Autodesk Inventor part; units mm, degrees
ref_plane "YZ Plane" through (0, 0, 0) normal (1, 0, 0) x (0, 1, 0)
ref_plane "XZ Plane" through (0, 0, 0) normal (0, 1, 0) x (-1, 0, 0)
ref_plane "XY Plane" through (0, 0, 0) normal (0, 0, 1) x (1, 0, 0)
sketch "Sketch1" plane through (0, 0, 0) normal (0, 0, 1) x (1, 0, 0)
  line L0 (-106.553, -66.04) -> (-3.175, -66.04)
  line L1 (0, -62.865) -> (0, -3.175)
  line L2 (-3.175, 0) -> (-106.553, 0)
  line L3 (-109.728, -3.175) -> (-109.728, -62.865)
  arc A0 (-106.553, 0) -> (-109.728, -3.175) centre (-106.553, -3.175) ccw
  arc A1 (0, -3.175) -> (-3.175, 0) centre (-3.175, -3.175) ccw
  arc A2 (-3.175, -66.04) -> (0, -62.865) centre (-3.175, -62.865) ccw
  arc A3 (-109.728, -62.865) -> (-106.553, -66.04) centre (-106.553, -62.865) ccw
  line L4 (-101.6, 0) -> (-8.128, 0)
  line L5 (-8.128, 0) -> (-8.128, -66.04)
  line L6 (-8.128, -66.04) -> (-101.6, -66.04)
  line L7 (-101.6, -66.04) -> (-101.6, 0)
  line L8 (-109.728, -33.02) -> (0, -33.02)
  line L9 (-101.6, -33.02) -> (-8.128, -33.02)
  point P0 (0, 0)
  point P1 (0, -66.04)
  point P2 (-109.728, 0)
  dimension "d0" = 109.728
  dimension "d1" = 66.04
  dimension "d2" = 3.175
  dimension "d3" = 93.472
  dimension "d4" = 66.04
revolve "Revolution1" add sketch "Sketch1" angle 360 about axis through (-109.728, -33.02, 0) along (1, 0, 0) contours L8 L3 A0 L2 L7 | L5 L2 A1 L1 L8
sketch "Sketch2" plane through (-101.6, -33.02, 0) normal (1, 0, 0) x (0, 0, -1)
  circle A0 centre (0, 0) radius 33.02
  circle A1 centre (0, 0) radius 33.02
  point P0 (0, 33.02)
extrude "Extrusion1" add sketch "Sketch2" along normal blind 93.6625
sketch "Sketch3" plane through (-109.728, -33.02, 0) normal (-1, 0, 0) x (0, 0, 1)
  circle A0 centre (12.281, -11.8451) radius 1.5537
  circle A1 centre (12.281, -11.8451) radius 3.203
  circle A2 centre (18.9602, -7.3205) radius 1.5537
  circle A3 centre (18.9602, -7.3205) radius 2.8009
  point P0 (0, 33.02)
extrude "Extrusion2" add sketch "Sketch3" along normal blind 1.27 contours A0
sketch "Sketch4" plane through (-109.728, -33.02, 0) normal (-1, 0, 0) x (0, 0, 1)
  circle A0 centre (17.6824, -8.7825) radius 1.5648
  point P0 (0, 33.02)
extrude "Extrusion3" add sketch "Sketch4" along normal blind 1.27
equation "\"BendRadius\" = Thickness"
equation "\"BendReliefWidth\" = Thickness"
equation "\"BendReliefDepth\" = 0.5 * Thickness"
equation "\"CornerReliefSize\" = 4 * Thickness"
equation "\"MinimumRemnant\" = 2 * Thickness"
equation "\"TransitionRadius\" = BendRadius"
equation "\"JacobiRadiusSize\" = BendRadius"
equation "\"GapSize\" = Thickness"
properties part number "cim motor"
Can you work these out from the model? Positions are in its coordinate system, mm. A direction names the side the tool comes from. Coordinates: 2 decimals unless noted, no trailing zeros. Loops run counter-clockwise (first coordinate to the right, second up) from the corner with the lowest first, then second, coordinate; pieces in that order, holes last. Notation, with made-up numbers: (-34, 44.25) -> (19, 44.25) arc R15 ccw to (19, 48.25) -> close; hole circle Ø4 at (-2, 59). An arc over 180 degrees is marked (long way). Put each result on its own line as item: value. Start each with the question number.
Q1. I want a section at A-A (x = -49). Write out the boundary of the cut face in (y, z).
Q2. Thinking about a two-plate mould opening in Y: for faces 3 (the face through (-110.354, -44.27, 13.716)), 4 (the face through (-109.728, -33, 0)), which applies, pulls with the +Y half, pulls with the -Y half, needs draft (parallel to the pull), parting line crosses it, or undercut?
Q3. If I drill on line 1 (X direction, y = -23, z = -5.5); line 2 (Z direction, x = -92.5, y = -62); line 3 (Z direction, x = -35, y = -27.5), over which ranges is the centre line in solid material (lowest first)? Write a range as [from, to].
Q4. For faces 1 (the face through (-110.35, -40.85, 16.44)), 2 (the face through (-110.998, -45, 12)), which set-ups out of +Z, -Z, +X, -X, +Y, -Y let a thin tool reach every point of the face, with its end or its side?
Q5. I'm going to push flat-ended pins straight in: P1, Ø6, axis at x = -93.5, y = -11, coming from the +Z side; P2, Ø6, axis at y = -55.5, z = 19.5, coming from the -X side; P3, Ø1, axis at x = -95, y = -17, coming from the +Z side; P4, Ø1, axis at x = -62, z = 0.5, coming from the +Y side. Where does each tip first touch, or does it pass through?
Taken from the geometry:
1. outline: circle Ø66.04 at (-33.02, 0)
2. face 3: parting line crosses it
2. face 4: needs draft
3. line 1: x = [-109.73, 0]
3. line 2: z = [-15.83, 15.83]
3. line 3: z = [-32.56, 32.56]
4. face 1: -X
4. face 2: +Z, -Z, -X, +Y, -Y
5. P1: stops at z = 26.99
5. P2: stops at x = -109.73
5. P3: stops at z = 29.15
5. P4: stops at y = 0
